Check sheet for the modelled part. Datum: model origin and axes. Units: mm. A direction names the side the tool comes from. Give positions to 0.01 mm unless a question says otherwise; leave off trailing zeros. Order: outer loops, then holes, each group sorted by start corner. A loop starts at its lowest first (then second) coordinate and runs counter-clockwise, first axis right, second up. Notation, with made-up numbers: (-28, -20.75) -> (-16, -20.75) arc R19 ccw to (-16, 7.25) -> close; hole circle Ø1 at (69.5, 59.25). An arc over 180 degrees is marked (long way). Answer in a Markdown table with one row per item. Add a question column.
(1) Thickness scan on L1, parallel to Y at x = -5.75, z = 32; L2, parallel to Z at x = -0.5, y = -3; L3, parallel to X at y = 1.5, z = 31. Record the ranges inside material, lowest first. Write a range as [from, to].
(2) Go/stop test with flat-tipped pins: pin 1 (1.5 mm diameter, centred on y = -7.5, z = 29.5, fed in from -X); pin 2 (5 mm diameter, centred on x = -5, z = 21, fed in from -Y); pin 3 (0.7 mm diameter, centred on y = -3, z = 37.5, fed in from +X). Record where each tip stops, or that it passes through.
(3) Set-up check for faces 1 (the face through (-9.5, -7, 32)), 2 (the face through (-2.948, 2.851, 42.286)), 3 (the face through (-1.5, 3, 38)): record each of +Z, -Z, +X, -X, +Y, -Y from which the full face is reachable in a straight line by a thin tool's end or side.
(4) Cross-section at D-D (x = -6.25). State how many separate pieces and enclosed holes the cut face has, then the cut area to 3 significant figures.
(5) Cross-section at B-B (z = 36). Record the cut outline in (x, y).
(6) Cross-section at C-C (z = 15). Record the cut outline in (x, y), then the cut area to 3 significant figures.
(7) Release check for a two-part mould opening along Y. For faces 4 (the face through (-6, -2.25, 21)), 5 (the face through (-1.248, 0, 17)), 6 (the face through (-8.124, -2.866, 25.257)) record: released by +Y, released by -Y, zero draft, split by the parting line, or undercut.
(8) Cross-section at A-A (x = -3.95). Record the cut outline in (y, z), then the cut area to 4 significant figures.
Solid Edge part; units mm, degrees
sketch "Sketch1" plane through (0, 0, 0) normal (0, -1, 0) x (1, 0, 0)
  line L0 (0, 0) -> (0, 35)
  line L1 (0, 35) -> (-1.5, 35)
  line L2 (-1.5, 40.05) -> (-1.5, 35)
  arc A0 (-1.5, 40.05) -> (-5.521359, 41.929716) centre (-3.95, 40.05) ccw
  line L3 (-5.521359, 41.929716) -> (-11.202722, 29.775325)
  arc A1 (-11.202722, 29.775325) -> (-11.483188, 24.110112) centre (-4.408345, 26.599409) ccw
  line L4 (-3, 0) -> (-11.483188, 24.110112)
  line L5 (0, 0) -> (-3, 0)
  circle A2 centre (-3.95, 40.05) radius 0.95
  circle A3 centre (-6.25, 15) radius 0.95
  circle A4 centre (-8, 26.199407) radius 0.95
extrude "Protrusion1" add sketch "Sketch1" along normal mid plane 7
sketch "Sketch2" plane through (-1.5, 0, 0) normal (0, 0, -1) x (0, 1, 0)
  line L0 (2.25, 0.251655) -> (-2.25, 0.251655)
  line L1 (-2.25, 0.251655) -> (-2.25, -10.408345)
  line L2 (2.25, -10.408345) -> (-2.25, -10.408345)
  line L3 (2.25, 0.251655) -> (2.25, -10.408345)
extrude "ExtrudedCutout_1" cut sketch "Sketch2" against normal blind 43.130726
fillet "Round_1" radius 0.5 4 edges at (0, 3.5, 17.5) (0, -3.5, 17.5) (-1.248345, -2.25, 17.5) (-1.248345, 2.25, 17.5)
sketch "Sketch3" plane through (-6.204172, -3.5, 21.25) normal (0, -1, 0) x (0.4234554, 0, 0.9059169)
  line L0 (5.35379, 4.484869) -> (5.883109, 3.352473)
  line L1 (5.883109, 3.352473) -> (9.053818, 4.834567)
  line L2 (9.053818, 4.834567) -> (7.99518, 7.099359)
  line L3 (7.99518, 7.099359) -> (4.824471, 5.617265)
  line L4 (4.824471, 5.617265) -> (5.35379, 4.484869)
extrude "ExtrudedProtrusion_3" add sketch "Sketch3" along normal blind 4 draft 10
sketch "Sketch4" plane through (-1.5, 0, 29.85) normal (0, 0, -1) x (1, 0, 0)
  line L0 (-8, 7.519768) -> (-8, 5.019768)
  spline S0 degree 3 poles (-8, 5.019768) (-7.628922, 5.044094) (-6.92286, 5.104892) (-5.68908, 5.582187) (-4.64629, 6.44206) (-4.261677, 7.116492) (-4.25, 7.519768) knots 0 0 0 0 0.211005 0.470829 0.806586 1 1 1 1
revolve "RevolvedProtrusion_2" add sketch "Sketch4" angle 360 about axis through (-9.5, -7.519768, 29.85) along (1, 0, 0)
sketch "Sketch5" plane through (-6.204172, -7.519768, 21.25) normal (0, -1, 0) x (0.4234554, 0, 0.9059169)
  line L0 (6.39525, 6.627463) -> (4.583416, 5.780552)
  arc A0 (6.501113, 6.400984) -> (4.583416, 5.780552) centre (3.060538, 13.761559) cw
revolve "RevolvedCutout1" cut sketch "Sketch5" angle 360 about axis through (-9.5, -7.519768, 29.85) along (1, 0, 0)
properties material "Stainless Steel, 420"
Answer below:
| question | item | result |
|---|---|---|
| 1 | L1 | y = [-3.5, -2.25], [2.25, 3.5] |
| 1 | L2 | z = [0, 35] |
| 1 | L3 | x = [-1.25, 0] |
| 2 | pin 1 | stops at x = -9.32 |
| 2 | pin 2 | stops at y = -3.5 |
| 2 | pin 3 | stops at x = -1.5 |
| 3 | face 1 | +Z, -Z, -X, -Y |
| 3 | face 2 | +Z, +Y, -Y |
| 3 | face 3 | +Z, +X, +Y, -Y |
| 4 | separate pieces | 5 |
| 4 | enclosed holes | 0 |
| 4 | area | 76.7 mm² |
| 5 | outline | (-8.29, -3.5) -> (-1.5, -3.5) -> (-1.5, -2.18) arc R0.5 cw to (-1.75, -2.25) -> (-8.29, -2.25) -> close; (-8.29, 2.25) -> (-1.75, 2.25) arc R0.5 cw to (-1.5, 2.18) -> (-1.5, 3.5) -> (-8.29, 3.5) -> close |
| 6 | outline | (-8.28, -3.5) -> (-7.2, -3.5) -> (-7.2, -2.25) -> (-8.28, -2.25) -> close; (-8.28, 2.25) -> (-7.2, 2.25) -> (-7.2, 3.5) -> (-8.28, 3.5) -> close; (-5.3, -3.5) -> (-0.5, -3.5) arc R0.5 ccw to (0, -3) -> (0, 3) arc R0.5 ccw to (-0.5, 3.5) -> (-5.3, 3.5) -> (-5.3, 2.25) -> (-1.75, 2.25) arc R0.5 cw to (-1.25, 1.75) -> (-1.25, -1.75) arc R0.5 cw to (-1.75, -2.25) -> (-5.3, -2.25) -> close |
| 6 | area | 21.6 mm² |
| 7 | face 4 | undercut |
| 7 | face 5 | undercut |
| 7 | face 6 | zero draft |
| 8 | outline | (-3.5, 2.7) -> (-2.25, 2.7) -> (-2.25, 39.1) -> (-3.5, 39.1) -> close; (-3.5, 41) -> (-2.25, 41) -> (-2.25, 42.5) -> (-3.5, 42.5) -> close; (2.25, 2.7) -> (3.5, 2.7) -> (3.5, 39.1) -> (2.25, 39.1) -> close; (2.25, 41) -> (3.5, 41) -> (3.5, 42.5) -> (2.25, 42.5) -> close |
| 8 | area | 94.75 mm² |
